Source: three-view drawing plus pictorial views. Frame: mm from the lowest corner of the part. A direction names the side the tool comes from. Round coordinates to 2 decimals unless told otherwise and drop trailing zeros. Order: outer loops, then holes, each group sorted by start corner. A loop starts at its lowest first (then second) coordinate and runs counter-clockwise, first axis right, second up. Notation, with made-up numbers: M 9.25,67.5 L 46.25,67.5 A13 cw 46.25,87.5 Z; hole C -39.75,74 d9. An arc over 180 degrees is marked long. Return JSON: item names as keys, results as strings. Group by question number.
Q1. Cut plane B-B on z = 15. Output: boundary loops of the cut face in (x, y), and give its area (3 significant figures).
Q2. Cut plane D-D on z = 3. Output: boundary loops of the cut face in (x, y).
Q3. Ray query, probe 1 along Y at (x, z) = (12.5, 13.5); probe 2 along Z at (x, y) = (11, 15.5); probe 3 along Z at (x, y) = (4, 19.75). Return the intervals inside material, ascending.
Q4. Cut plane A-A on x = 12.5. Output: boundary loops of the cut face in (y, z), and give its area (3 significant figures).
Q5. Access query for the marked faces 1 and 2. Directions: +Z, -Z, +X, -X, +Y, -Y. A direction counts if a zero-diameter tool reaches every point of the face in a straight line with its end or side. Return the directions, or none.
Q6. Cut plane C-C on y = 12.5. Output: boundary loops of the cut face in (x, z), and give its area (3 significant figures).
Q7. Contact query for flat-ended pins moving along their axis: pin 1 (1.5 mm diameter, centred on x = 15.5, y = 17.5, fed in from +Z); pin 2 (3 mm diameter, centred on x = 19, z = 14.5, fed in from -Y); pin 3 (4 mm diameter, centred on y = 21.5, z = 9, fed in from +X); pin 4 (4 mm diameter, centred on y = 6.5, z = 24.5, fed in from +X). Output: stop coordinate, or through.
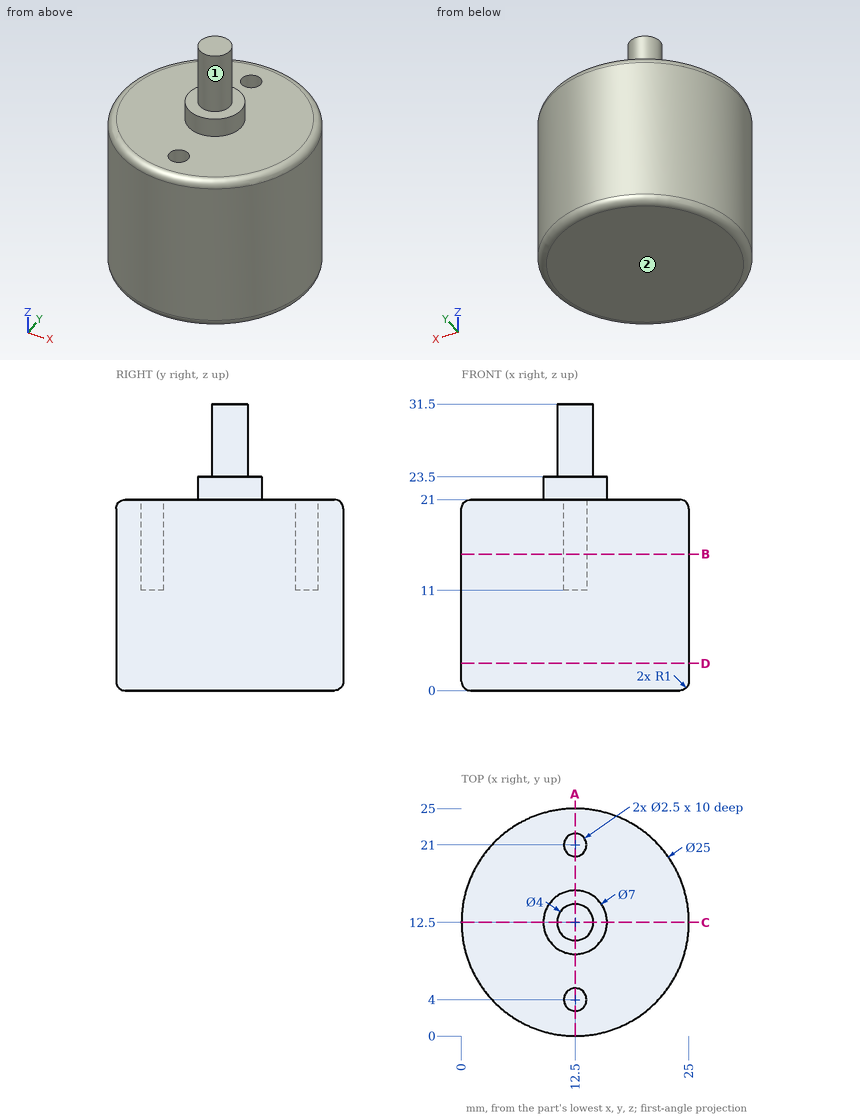
Result sheet:
{
 "1": {"outline": "C 12.5,12.5 d25; hole C 12.5,4 d2.5; hole C 12.5,21 d2.5", "area": "481 mm²"},
 "2": {"outline": "C 12.5,12.5 d25"},
 "3": {"probe 1": "y = 0 to 2.75, 5.25 to 19.75, 22.25 to 25", "probe 2": "z = 0 to 23.5", "probe 3": "z = 0 to 21"},
 "4": {"outline": "M 0,1 A1 ccw 1,0 L 24,0 A1 ccw 25,1 L 25,20 A1 ccw 24,21 L 22.25,21 L 22.25,11 L 19.75,11 L 19.75,21 L 16,21 L 16,23.5 L 14.5,23.5 L 14.5,31.5 L 10.5,31.5 L 10.5,23.5 L 9,23.5 L 9,21 L 5.25,21 L 5.25,11 L 2.75,11 L 2.75,21 L 1,21 A1 ccw 0,20 Z", "area": "524 mm²"},
 "5": {"face 1": "+Z", "face 2": "-Z, +X, -X, +Y, -Y"},
 "6": {"outline": "M 0,1 A1 ccw 1,0 L 24,0 A1 ccw 25,1 L 25,20 A1 ccw 24,21 L 16,21 L 16,23.5 L 14.5,23.5 L 14.5,31.5 L 10.5,31.5 L 10.5,23.5 L 9,23.5 L 9,21 L 1,21 A1 ccw 0,20 Z", "area": "574 mm²"},
 "7": {"pin 1": "stops at z = 21", "pin 2": "stops at y = 1.04", "pin 3": "stops at x = 22.86", "pin 4": "passes through"}
}
